The model under review builds one solid part; all positions refer to its coordinate system, in mm. Face numbers are marked on the shaded views. Round coordinates to 2 decimals unless told otherwise and drop trailing zeros. Order: outer loops, then holes, each group sorted by start corner. A loop starts at its lowest first (then second) coordinate and runs counter-clockwise, first axis right, second up. Notation, with made-up numbers: (-4.75, -39.75) - (39.25, -39.75) arc R18 cw to (39.25, -25.75) - close; hole circle Ø1 at (-21, 56.25). An arc over 180 degrees is marked (long way). One line per question, with ' | ' between items. Start each with the question number.
Item 1: Add section B-B on x = -10. State the section outline as (y, z) points.
Item 2: For L1, parallel to Z at x = 0, y = 154; L2, parallel to X at y = 37, z = -1; L3, parallel to Z at x = -13.5, y = 294.5, list the stretches that pass through material, from the lowest coordinate up. Write a range as [from, to].
Item 3: Insertion check: pin 1 Ø10 at (y, z) = (93, 7) entering from +X; pin 2 Ø1 at (y, z) = (225, 8) entering from -X; pin 3 Ø6 at (y, z) = (343, 8) entering from -X. Each pin has a flat end and moves straight along its axis. Give the tip position at first contact, or say it passes through.
Item 4: Add section A-A on z = 0. State the section outline as (x, y) points, and give its area (3 significant figures).
Item 5: Add section C-C on y = 246. State the section outline as (x, z) points.
Item 6: Draft analysis for pull direction Z (two halves, no side actions). For the marked faces 1 and 2, state which applies: +Z half, -Z half, draft (parallel to the pull), parting line (faces both ways), or undercut.
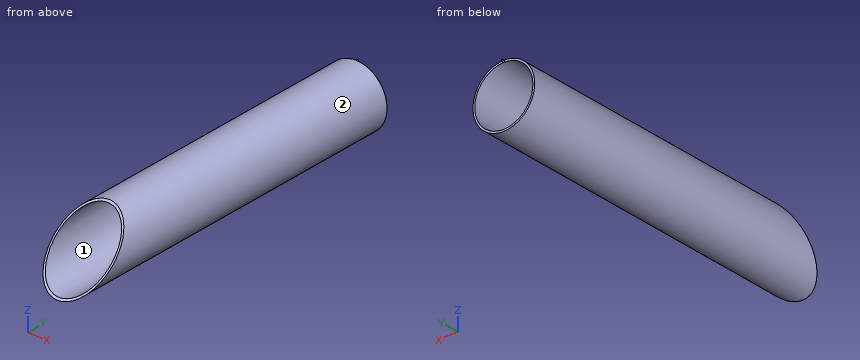
Autodesk Inventor part; units mm, degrees
ref_plane "YZ Plane" through (0, 0, 0) normal (1, 0, 0) x (0, 1, 0)
ref_plane "XZ Plane" through (0, 0, 0) normal (0, 1, 0) x (-1, 0, 0)
ref_plane "XY Plane" through (0, 0, 0) normal (0, 0, 1) x (1, 0, 0)
sketch "Sketch1" plane through (0, 0, 0) normal (0, 1, 0) x (-1, 0, 0)
  circle A0 centre (0, 0) radius 35
  circle A1 centre (0, 0) radius 33
  dimension "d0" = 2
  dimension "d1" = 70
extrude "Extrusion1" add sketch "Sketch1" along normal blind 400
sketch "Sketch2" plane through (0, 0, 0) normal (1, 0, 0) x (0, 1, 0)
  line L0 (0, -35) -> (0, 35)
  line L1 (0, -35) -> (70, 35)
  line L2 (0, 35) -> (400, 35)
  point P0 (0, 0)
  dimension "d4" = 70
extrude "Extrusion2" cut sketch "Sketch2" along normal through all both and the other way through all
sketch "Sketch4" plane through (0, 400, 0) normal (0, 1, 0) x (1, 0, 0)
  circle A0 centre (0, -34) radius 1
  circle A1 centre (0, 0) radius 33
  circle A2 centre (0, 0) radius 35
extrude "Extrusion4" add sketch "Sketch4" along normal blind 2 contours A0
properties part number "Feul_Intake"
Determined:
1) outline: (1.46, -33.54) - (400, -33.54) - (400, -31.45) - (3.55, -31.45) - close; (66.45, 31.45) - (400, 31.45) - (400, 33.54) - (68.54, 33.54) - close
2) L1: [-35, -33], [33, 35] | L2: [-34.99, -32.98], [32.98, 34.99] | L3: [-32.29, -30.11], [30.11, 32.29]
3) pin 1: x = 34.94 | pin 2: x = -34.19 | pin 3: x = -34.64
4) outline: (-35, 35) - (-33, 35) - (-33, 400) - (-35, 400) - close; (33, 35) - (35, 35) - (35, 400) - (33, 400) - close | area: 1,460 mm2
5) outline: circle Ø70 at (0, 0); hole circle Ø66 at (0, 0)
6) face 1: undercut | face 2: parting line
